Work out the finished part from the listing and answer in its coordinate system (mm). Round coordinates to 2 decimals unless told otherwise and drop trailing zeros. Write each loop counter-clockwise with the first axis right and the second up, starting at its lowest first coordinate (ties: lowest second). Pieces come first, ordered by that corner, then holes.
1. Find section A-A (y = 0). Write down the section's boundary in (x, z), and give its area (3 significant figures).
2. Determine the mould class of faces 1 (the face through (11, 1, 5)), 2 (the face through (0, 0, 5)), 3 (the face through (-0.596, 2.685, 7.465)), 4 (the face through (-1.08, 4.88, 8.48)) for opening direction X: pulls with the +X half, pulls with the -X half, needs draft (parallel to the pull), parting line crosses it, or undercut.
3. Flat-ended cylindrical pins translate along their axes: pin 1 Ø3 at (x, y) = (1, 0) entering from +Z; pin 2 Ø3 at (x, z) = (-22, 8) entering from -Y; pin 3 Ø1 at (x, z) = (-38, 2) entering from +Y. Find the tip coordinate at first contact, or state that the pin passes through.
4. Straight lines are drawn through the part: probe 1 along Y at (x, z) = (0, 7); probe 2 along Z at (x, y) = (24, -20); probe 3 along Y at (x, z) = (0, 6.6). For each, find the intervals that lie inside material, in ascending order.
5. Find section C-C (y = 39). Write down the section's boundary in (x, z).
6. Find section D-D (x = -37.5). Write down the section's boundary in (y, z), and give its area (3 significant figures).
Autodesk Inventor part; units mm, degrees
ref_plane "YZ Plane" through (0, 0, 0) normal (1, 0, 0) x (0, 1, 0)
ref_plane "XZ Plane" through (0, 0, 0) normal (0, 1, 0) x (-1, 0, 0)
ref_plane "XY Plane" through (0, 0, 0) normal (0, 0, 1) x (1, 0, 0)
sketch "Sketch4" plane through (0, 0, 0) normal (0, 0, 1) x (1, 0, 0)
  circle A0 centre (0, 0) radius 51.25
  circle A1 centre (0, 0) radius 2.75
  dimension "d10" = 102.5
  dimension "d11" = 5.5
extrude "Extrusion4" add sketch "Sketch4" along normal blind 5
sketch "Sketch5" plane through (0, 0, 5) normal (0, 0, 1) x (1, 0, 0)
  circle A0 centre (0, 0) radius 2.75
  circle A1 centre (0, 0) radius 2.75
  circle A2 centre (0, 0) radius 5
  dimension "d14" = 10
extrude "Extrusion5" add sketch "Sketch5" along normal blind 5
chamfer "Chamfer1" distance 2 angle 45 1 edges at (-5, 0, 5)
sketch "Sketch6" plane through (0, 0, 0) normal (0, 0, -1) x (-1, 0, 0)
  circle A0 centre (0, 0) radius 2.75
  circle A1 centre (0, 0) radius 2.75
extrude "Extrusion6" add sketch "Sketch6" against normal blind 5
sketch "Sketch7" plane through (0, 0, 0) normal (0, 0, -1) x (-1, 0, 0)
  point P0 (0, 0)
properties part number "bottom"
Worked answers:
1. outline: (-51.25, 0) - (51.25, 0) - (51.25, 5) - (7, 5) - (5, 7) - (5, 10) - (2.75, 10) - (2.75, 5) - (-2.75, 5) - (-2.75, 10) - (-5, 10) - (-5, 7) - (-7, 5) - (-51.25, 5) - close
1. area: 539 mm2
2. face 1: needs draft
2. face 2: undercut
2. face 3: undercut
2. face 4: parting line crosses it
3. pin 1: stops at z = 5
3. pin 2: passes through
3. pin 3: stops at y = 34.93
4. probe 1: y = -5 to -2.75, 2.75 to 5
4. probe 2: z = 0 to 5
4. probe 3: y = -5.4 to -2.75, 2.75 to 5.4
5. outline: (-33.25, 0) - (33.25, 0) - (33.25, 5) - (-33.25, 5) - close
6. outline: (-34.93, 0) - (34.93, 0) - (34.93, 5) - (-34.93, 5) - close
6. area: 349 mm2
